Autodesk Fusion 360 part; units mm, degrees
sketch "Sketch1" plane through (0, 0, 0) normal (0, 1, 0) x (1, 0, 0)
  circle A0 centre (0, 0) radius 10
  circle A1 centre (0, 0) radius 20
  circle A2 centre (0, 0) radius 18.0278 construction
  circle A3 centre (-0.0049, -16.3778) radius 1.65
  line L0 (0, -22) -> (0, 22) construction
  line L1 (-25, 0) -> (28, 0) construction
  circle A4 centre (0, 0) radius 10
  circle A5 centre (0, 0) radius 10
  circle A6 centre (14.1811, -8.1931) radius 1.65
  circle A7 centre (14.186, 8.1846) radius 1.65
  circle A8 centre (0.0049, 16.3778) radius 1.65
  circle A9 centre (-14.1811, 8.1931) radius 1.65
  circle A10 centre (-14.186, -8.1846) radius 1.65
  point P0 (-0.0049, -16.3778)
  point P1 (-0.0049, 16.3778)
  dimension "d1" = 20
  dimension "d2" = 40
  dimension "d3" = 3.3
  dimension "d16" = 360
extrude "Extrude1" add sketch "Sketch1" along normal blind 13 contours A0 A4 A5 | A1 | A3 | A6 | A7 | A8 | A9 | A10
extrude "Extrude3" cut sketch "Sketch1" along normal blind 3 contours A0 A4 A5
fillet "Fillet1" radius 1.5 2 edges at (-18.6465, 0, 7.2323) (-18.6465, 13, 7.2323)
extrude "Extrude4" cut sketch "Sketch1" along normal blind 8 contours A3 | A6 | A7 | A8 | A9 | A10
sketch "Sketch2" plane through (0, 13, 0) normal (0, 1, 0) x (-1, 0, 0)
  circle A0 centre (0, 0) radius 18.5
  circle A1 centre (0, 0) radius 18
  dimension "d17" = 36
extrude "Extrude5" cut sketch "Sketch2" against normal blind 3 contours A1
Source: CAD feature listing. Evaluate the final solid. Frame: model axes, mm. A direction names the side the tool comes from. Give positions to 0.01 mm unless a question says otherwise; leave off trailing zeros. Write each loop counter-clockwise with the first axis right and the second up, starting at its lowest first coordinate (ties: lowest second). Pieces come first, ordered by that corner, then holes.
1. Section query B-B (y = 3.5). Return the cut outline in (x, z).
2. Access query for faces 1 (the face through (8, 0, 8)), 2 (the face through (14, 8, -8)), 3 (the face through (2.343, 11.521, 17.847)). Directions: +Z, -Z, +X, -X, +Y, -Y. A direction counts if a zero-diameter tool reaches every point of the face in a straight line with its end or side. Return the directions, or none.
3. Section query D-D (y = 10.75). Return the cut outline in (x, z).
4. Pull-direction query (Z, two-part tool) for faces 4 (the face through (0, 8, -16)), 5 (the face through (-4.336, 6.43, -19.524)), 6 (the face through (4.02, 13, 17.73)); classes: +Z half, -Z half, draft (parallel to the pull), parting line (faces both ways), or undercut.
5. Section query C-C (z = 0). Return the cut outline in (x, y).
6. Material intervals for line 1 along X through (y, z) = (1.6, 0); line 2 along X through (y, z) = (3.5, 9); line 3 along Y through (x, z) = (-16.5, -2), sorted ascending.
7. Section query A-A (x = 0). Return the cut outline in (y, z), then the cut area to 3 significant figures.
8. First-contact query: pin 1 (6 mm diameter, centred on y = 11, z = 12, fed in from -X); pin 2 (2 mm diameter, centred on x = 14.18, z = 8.19, fed in from -Y); pin 3 (16 mm diameter, centred on x = 0, z = 0, fed in from -Y). Flat tips, straight axial feed; report the tip coordinate or a pass-through.
Output values:
1. outline: circle Ø40 at (0, 0); hole circle Ø3.3 at (-14.19, 8.18); hole circle Ø3.3 at (-14.18, -8.19); hole circle Ø3.3 at (0, -16.38); hole circle Ø3.3 at (0, 16.38); hole circle Ø3.3 at (14.18, 8.19); hole circle Ø3.3 at (14.19, -8.18)
2. face 1: +Z, -Z, +X, -X, -Y
2. face 2: -Y
2. face 3: +Y
3. outline: circle Ø40 at (0, 0); hole circle Ø36 at (0, 0)
4. face 4: undercut
4. face 5: parting line
4. face 6: draft
5. outline: (-20, 1.5) arc R1.5 ccw to (-18.5, 0) - (-10, 0) - (-10, 3) - (10, 3) - (10, 0) - (18.5, 0) arc R1.5 ccw to (20, 1.5) - (20, 11.5) arc R1.5 ccw to (18.5, 13) - (18, 13) - (18, 10) - (-18, 10) - (-18, 13) - (-18.5, 13) arc R1.5 ccw to (-20, 11.5) - close
6. line 1: x = -20 to -10, 10 to 20
6. line 2: x = -17.86 to -15.62, -12.75 to 12.74, 15.62 to 17.86
6. line 3: y = 0 to 10
7. outline: (0, -18.5) arc R1.5 ccw to (1.5, -20) - (11.5, -20) arc R1.5 ccw to (13, -18.5) - (13, -18) - (10, -18) - (10, 18) - (13, 18) - (13, 18.5) arc R1.5 ccw to (11.5, 20) - (1.5, 20) arc R1.5 ccw to (0, 18.5) - (0, 18.03) - (8, 18.03) - (8, 14.73) - (0, 14.73) - (0, 10) - (3, 10) - (3, -10) - (0, -10) - (0, -14.73) - (8, -14.73) - (8, -18.03) - (0, -18.03) - close
7. area: 297 mm2
8. pin 1: stops at x = -17.86
8. pin 2: stops at y = 8
8. pin 3: stops at y = 3
